The listing builds one solid part. Answer for the finished solid, in the listing's coordinates (mm). A direction names the side the tool comes from. Give positions to 0.01 mm unless a question says otherwise; leave off trailing zeros. Loops run counter-clockwise (first coordinate to the right, second up) from the corner with the lowest first, then second, coordinate; pieces in that order, holes last. Notation, with made-up numbers: (12, -18) - (46, -18) arc R11 cw to (46, -5) - close; hole circle Ø11 at (6, -27). An arc over 180 degrees is marked (long way). One line per item, written item: value. Start each with the question number.
from build123d import *

# Parameters (mm, degrees)
F1_DEPTH = 30


with BuildPart() as f1:
    # F0 (on Front) → F1 (new body)
    with BuildSketch(Plane.XZ):
        with BuildLine():
            Line((211.123637, 0), (211.123637, 80))
            ThreePointArc((211.123637, 80), (208.194705, 87.071068), (201.123637, 90))
            Line((201.123637, 90), (21.123637, 90))
            ThreePointArc((21.123637, 90), (14.052569, 92.928932), (11.123637, 100))
            Line((11.123637, 100), (11.123637, 110))
            ThreePointArc((11.123637, 110), (8.194705, 117.071068), (1.123637, 120))
            Line((1.123637, 120), (-98.876363, 120))
            ThreePointArc((-98.876363, 120), (-105.947431, 117.071068), (-108.876363, 110))
            Line((-108.876363, 110), (-108.876363, -30))
            ThreePointArc((-108.876363, -30), (-105.947431, -37.071068), (-98.876363, -40))
            Line((-98.876363, -40), (1.123637, -40))
            ThreePointArc((1.123637, -40), (8.194705, -37.071068), (11.123637, -30))
            Line((11.123637, -30), (11.123637, -20))
            ThreePointArc((11.123637, -20), (14.052569, -12.928932), (21.123637, -10))
            Line((21.123637, -10), (201.123637, -10))
            ThreePointArc((201.123637, -10), (208.194705, -7.071068), (211.123637, 0))
        make_face()
        with BuildLine():
            ThreePointArc((-88.876363, 10), (-85.947431, 17.071068), (-78.876363, 20))
            Line((-78.876363, 20), (-18.876363, 20))
            ThreePointArc((-18.876363, 20), (-11.805295, 17.071068), (-8.876363, 10))
            Line((-8.876363, 10), (-8.876363, -10))
            ThreePointArc((-8.876363, -10), (-11.805295, -17.071068), (-18.876363, -20))
            Line((-18.876363, -20), (-78.876363, -20))
            ThreePointArc((-78.876363, -20), (-85.947431, -17.071068), (-88.876363, -10))
            Line((-88.876363, -10), (-88.876363, 10))
        make_face(mode=Mode.SUBTRACT)
        with BuildLine():
            ThreePointArc((15.246786, 10), (18.175718, 17.071068), (25.246786, 20))
            Line((25.246786, 20), (180.47985, 20))
            ThreePointArc((180.47985, 20), (187.550918, 17.071068), (190.47985, 10))
            ThreePointArc((190.47985, 10), (187.550918, 2.928932), (180.47985, 0))
            Line((180.47985, 0), (25.246786, 0))
            ThreePointArc((25.246786, 0), (18.175718, 2.928932), (15.246786, 10))
        make_face(mode=Mode.SUBTRACT)
        with BuildLine():
            ThreePointArc((-88.876363, 90), (-85.947431, 97.071068), (-78.876363, 100))
            Line((-78.876363, 100), (-18.876363, 100))
            ThreePointArc((-18.876363, 100), (-11.805295, 97.071068), (-8.876363, 90))
            Line((-8.876363, 90), (-8.876363, 70))
            ThreePointArc((-8.876363, 70), (-11.805295, 62.928932), (-18.876363, 60))
            Line((-18.876363, 60), (-78.876363, 60))
            ThreePointArc((-78.876363, 60), (-85.947431, 62.928932), (-88.876363, 70))
            Line((-88.876363, 70), (-88.876363, 90))
        make_face(mode=Mode.SUBTRACT)
        with BuildLine():
            ThreePointArc((16.214924, 40), (19.143856, 47.071068), (26.214924, 50))
            Line((26.214924, 50), (181.447988, 50))
            ThreePointArc((181.447988, 50), (188.519056, 47.071068), (191.447988, 40))
            ThreePointArc((191.447988, 40), (188.519056, 32.928932), (181.447988, 30))
            Line((181.447988, 30), (26.214924, 30))
            ThreePointArc((26.214924, 30), (19.143856, 32.928932), (16.214924, 40))
        make_face(mode=Mode.SUBTRACT)
        with BuildLine():
            ThreePointArc((16.214924, 70), (19.143856, 77.071068), (26.214924, 80))
            Line((26.214924, 80), (181.447988, 80))
            ThreePointArc((181.447988, 80), (188.519056, 77.071068), (191.447988, 70))
            ThreePointArc((191.447988, 70), (188.519056, 62.928932), (181.447988, 60))
            Line((181.447988, 60), (26.214924, 60))
            ThreePointArc((26.214924, 60), (19.143856, 62.928932), (16.214924, 70))
        make_face(mode=Mode.SUBTRACT)
    extrude(amount=F1_DEPTH)


solid = f1.part
1. A cutting plane is placed at C-C (y = -25.5). Give the number of separate pieces and of enclosed holes in the cut face, plus the area to 3 significant figures.
2. Determine the mould class of faces 3 (the flat face through (-88.876, -15, 0)), 4 (the flat face through (103, -15, 50)), 5 (the flat face through (13, -30, 41)), 6 (the cylindrical face through (8.272, -14.79, 116.993)) for opening direction Z: released by +Z, released by -Z, zero draft, split by the parting line, or undercut.
3. Flat-ended cylindrical pins translate along their axes: pin 1 (5 mm diameter, centred on y = -8, z = -27, fed in from +X); pin 2 (15 mm diameter, centred on x = 89, y = -17, fed in from -Z); pin 3 (10 mm diameter, centred on x = 97.5, y = -14.5, fed in from +Z). Find the tip coordinate at first contact, or state that the pin passes through.
4. For faces 1 (the cylindrical face through (-105.87, -14.79, 117.15)), 2 (the flat face through (-49, -15, 100)), determine the directions among +Z, -Z, +X, -X, +Y, -Y from which every point of the face is accessible in a straight line to the end or side of a thin tool.
5. A cutting plane is placed at A-A (x = -73). Determine the outline of the cut face in (y, z).
6. Find the intervals of material crossed by L1, parallel to Z at x = 120, y = -26.5; L2, parallel to Z at x = -48, y = -22.25; L3, parallel to X at y = -25.5, z = 66, in increasing order. Write a range as [from, to].
7. A cutting plane is placed at B-B (x = 63.5). Determine the outline of the cut face in (y, z).
Results below:
1. separate pieces: 1
1. enclosed holes: 5
1. area: 22,600 mm^2
2. face 3: undercut
2. face 4: undercut
2. face 5: zero draft
2. face 6: released by +Z
3. pin 1: stops at x = 11.12
3. pin 2: stops at z = -10
3. pin 3: stops at z = 90
4. face 1: +Z, -X, +Y, -Y
4. face 2: +Y, -Y
5. outline: (-30, -40) - (0, -40) - (0, -20) - (-30, -20) - close; (-30, 20) - (0, 20) - (0, 60) - (-30, 60) - close; (-30, 100) - (0, 100) - (0, 120) - (-30, 120) - close
6. L1: z = [-10, 0], [20, 30], [50, 60], [80, 90]
6. L2: z = [-40, -20], [20, 60], [100, 120]
6. L3: x = [-108.88, -88.04], [-9.71, 17.05], [190.61, 211.12]
7. outline: (-30, -10) - (0, -10) - (0, 0) - (-30, 0) - close; (-30, 20) - (0, 20) - (0, 30) - (-30, 30) - close; (-30, 50) - (0, 50) - (0, 60) - (-30, 60) - close; (-30, 80) - (0, 80) - (0, 90) - (-30, 90) - close
